from build123d import *

# Parameters (mm, degrees)
SKETCH1_W           = 115
SKETCH1_H           = 115
SKETCH1_R           = 2.6
BOSS_EXTRUDE1_DEPTH = 2
SKETCH2_R           = 2.1
CUT_EXTRUDE1_DEPTH  = 82.341871137
SKETCH3_W           = 17.5
SKETCH3_H           = 22.5
CUT_EXTRUDE2_DEPTH  = 82.341871137
SKETCH4_R           = 1.6
CUT_EXTRUDE3_DEPTH  = 82.341871137
CUT_EXTRUDE4_DEPTH  = 82.341871137
SKETCH7_W           = 17.5
SKETCH7_H           = 22.5
BOSS_EXTRUDE2_DEPTH = 2
FILLET1_R           = 1.5


with BuildPart() as part:
    # Sketch1 → Boss-Extrude1 (new body)
    with BuildSketch(Plane(origin=(0, 0, 0), x_dir=(1, 0, 0), z_dir=(0, 1, 0))):
        Rectangle(SKETCH1_W, SKETCH1_H)
        with Locations(Location((-37.5, 45, 0), (0, 0, 270))):
            Circle(SKETCH1_R, mode=Mode.SUBTRACT)
        with Locations(Location((37.5, 45, 0), (0, 0, 90))):
            Circle(SKETCH1_R, mode=Mode.SUBTRACT)
        with Locations(Location((37.5, -45, 0), (0, 0, 270))):
            Circle(SKETCH1_R, mode=Mode.SUBTRACT)
        with Locations(Location((-37.5, -45, 0), (0, 0, 90))):
            Circle(SKETCH1_R, mode=Mode.SUBTRACT)
    extrude(amount=BOSS_EXTRUDE1_DEPTH)

    # Sketch2 → Cut-Extrude1 (cut, through all)
    with BuildSketch(Plane(origin=(0, 2, 0), x_dir=(1, 0, 0), z_dir=(0, 1, 0))):
        with Locations(Location((-49.5, -32, 0), (0, 0, 270))):
            Circle(SKETCH2_R)
        with Locations(Location((-25.5, -32, 0), (0, 0, 90))):
            Circle(SKETCH2_R)
        with Locations(Location((-25.5, -50, 0), (0, 0, 270))):
            Circle(SKETCH2_R)
        with Locations(Location((-49.5, -50, 0), (0, 0, 90))):
            Circle(SKETCH2_R)
        with Locations(Location((25.5, -50, 0), (0, 0, 90))):
            Circle(SKETCH2_R)
        with Locations(Location((49.5, -50, 0), (0, 0, 270))):
            Circle(SKETCH2_R)
        with Locations(Location((49.5, -32, 0), (0, 0, 90))):
            Circle(SKETCH2_R)
        with Locations(Location((25.5, -32, 0), (0, 0, 270))):
            Circle(SKETCH2_R)
        with Locations(Location((49.5, 50, 0), (0, 0, 90))):
            Circle(SKETCH2_R)
        with Locations(Location((49.5, 32, 0), (0, 0, 270))):
            Circle(SKETCH2_R)
        with Locations(Location((25.5, 50, 0), (0, 0, 270))):
            Circle(SKETCH2_R)
        with Locations(Location((25.5, 32, 0), (0, 0, 90))):
            Circle(SKETCH2_R)
        with Locations(Location((-25.5, 50, 0), (0, 0, 90))):
            Circle(SKETCH2_R)
        with Locations(Location((-49.5, 50, 0), (0, 0, 270))):
            Circle(SKETCH2_R)
        with Locations(Location((-49.5, 32, 0), (0, 0, 90))):
            Circle(SKETCH2_R)
        with Locations(Location((-25.5, 32, 0), (0, 0, 270))):
            Circle(SKETCH2_R)
    extrude(amount=-CUT_EXTRUDE1_DEPTH, mode=Mode.SUBTRACT)

    # Sketch3 → Cut-Extrude2 (cut, through all)
    with BuildSketch(Plane(origin=(0, 2, 0), x_dir=(1, 0, 0), z_dir=(0, 1, 0))):
        with Locations((0, -46.25)):
            Rectangle(SKETCH3_W, SKETCH3_H)
    extrude(amount=-CUT_EXTRUDE2_DEPTH, mode=Mode.SUBTRACT)

    # Sketch4 → Cut-Extrude3 (cut, through all)
    with BuildSketch(Plane(origin=(0, 2, 0), x_dir=(1, 0, 0), z_dir=(0, 1, 0))):
        with Locations(Location((-11.075, 49.5, 0), (0, 0, 270))):
            Circle(SKETCH4_R)
        with Locations(Location((11.075, 49.5, 0), (0, 0, 90))):
            Circle(SKETCH4_R)
    extrude(amount=-CUT_EXTRUDE3_DEPTH, mode=Mode.SUBTRACT)

    # Sketch6 → Cut-Extrude4 (cut, through all)
    with BuildSketch(Plane(origin=(0, 2, 0), x_dir=(1, 0, 0), z_dir=(0, 1, 0))):
        with BuildLine():
            Line((-34.9, 47.5), (-34.9, 42.5))
            ThreePointArc((-34.9, 42.5), (-37.5, 39.9), (-40.1, 42.5))
            Line((-40.1, 42.5), (-40.1, 47.5))
            ThreePointArc((-40.1, 47.5), (-37.5, 50.1), (-34.9, 47.5))
        make_face()
        with BuildLine():
            Line((34.9, 47.5), (34.9, 42.5))
            ThreePointArc((34.9, 42.5), (37.5, 39.9), (40.1, 42.5))
            Line((40.1, 42.5), (40.1, 47.5))
            ThreePointArc((40.1, 47.5), (37.5, 50.1), (34.9, 47.5))
        make_face()
    extrude(amount=-CUT_EXTRUDE4_DEPTH, mode=Mode.SUBTRACT)

    # Sketch7 → Boss-Extrude2 (add, through all)
    with BuildSketch(Plane(origin=(0, 2, 0), x_dir=(1, 0, 0), z_dir=(0, 1, 0))):
        with Locations((0, -46.25)):
            Rectangle(SKETCH7_W, SKETCH7_H)
    extrude(amount=-BOSS_EXTRUDE2_DEPTH)

    # Fillet1
    fillet1_edges = [part.edges().sort_by_distance(p)[0] for p in [
        (57.5, 1, 57.5),
        (-57.5, 1, 57.5),
        (-57.5, 1, -57.5),
        (57.5, 1, -57.5),
    ]]
    fillet(fillet1_edges, radius=FILLET1_R)


solid = part.part
Read the model definition and answer for the solid it produces. Units are mm, in the model's axes. Round coordinates to 2 decimals unless told otherwise and drop trailing zeros. Order: outer loops, then holes, each group sorted by start corner. A loop starts at its lowest first (then second) coordinate and runs counter-clockwise, first axis right, second up. Notation, with made-up numbers: (-17, -38.75) - (23, -38.75) arc R29 ccw to (23, -7.75) - close; hole circle Ø11 at (87, -33.75). An arc over 180 degrees is marked (long way). Use one line per item in the form item = value. Start each with the question number.
(1) The part is cut by section C-C (x = -37.5). Give the vertices of the cut face in (y, z), then the cut area to 3 significant figures.
(2) Flat-ended cylindrical pins translate along their axes: pin 1 Ø10 at (x, z) = (-38.5, 21) entering from -Y; pin 2 Ø4 at (x, z) = (25.5, -32) entering from -Y. Find the tip coordinate at first contact, or state that the pin passes through.
(3) The part is cut by section D-D (z = 50). Give the vertices of the cut face in (x, y).
(4) Find the intervals of material crossed by line 1 along X through (y, z) = (1.1, 50); line 2 along Z through (x, y) = (39.5, 1.5); line 3 along Z through (x, y) = (24, 0.8), in increasing order. Write a range as from..to.
(5) The part is cut by section A-A (x = 49.5). Give the vertices of the cut face in (y, z), then the cut area to 3 significant figures.
(6) The part is cut by section B-B (z = -45.5). Give the vertices of the cut face in (x, y).
Checked values:
q1.outline = (0, -57.5) - (2, -57.5) - (2, -50.1) - (0, -50.1) - close; (0, -39.9) - (2, -39.9) - (2, 42.4) - (0, 42.4) - close; (0, 47.6) - (2, 47.6) - (2, 57.5) - (0, 57.5) - close
q1.area = 199 mm^2
q2.pin_1 = 0
q2.pin_2 = through
q3.outline = (-57.5, 0) - (-51.6, 0) - (-51.6, 2) - (-57.5, 2) - close; (-47.4, 0) - (-27.6, 0) - (-27.6, 2) - (-47.4, 2) - close; (-23.4, 0) - (23.4, 0) - (23.4, 2) - (-23.4, 2) - close; (27.6, 0) - (47.4, 0) - (47.4, 2) - (27.6, 2) - close; (51.6, 0) - (57.5, 0) - (57.5, 2) - (51.6, 2) - close
q4.line_1 = -57.5..-51.6, -47.4..-27.6, -23.4..23.4, 27.6..47.4, 51.6..57.5
q4.line_2 = -57.5..-49.16, -40.84..43.34, 46.66..57.5
q4.line_3 = -57.5..-51.47, -48.53..-33.47, -30.53..30.53, 33.47..48.53, 51.47..57.5
q5.outline = (0, -57.5) - (2, -57.5) - (2, -52.1) - (0, -52.1) - close; (0, -47.9) - (2, -47.9) - (2, -34.1) - (0, -34.1) - close; (0, -29.9) - (2, -29.9) - (2, 29.9) - (0, 29.9) - close; (0, 34.1) - (2, 34.1) - (2, 47.9) - (0, 47.9) - close; (0, 52.1) - (2, 52.1) - (2, 57.5) - (0, 57.5) - close
q5.area = 196 mm^2
q6.outline = (-57.5, 0) - (-40.1, 0) - (-40.1, 2) - (-57.5, 2) - close; (-34.9, 0) - (34.9, 0) - (34.9, 2) - (-34.9, 2) - close; (40.1, 0) - (57.5, 0) - (57.5, 2) - (40.1, 2) - close
